Input: dimensioned drawing with shaded views. Units: mm. Origin: part minimum x, y, z. A direction names the side the tool comes from. Give positions to 0.01 mm unless a question says otherwise; leave off trailing zeros. Order: outer loops, then holes, each group sorted by start corner. A loop starts at its lowest first (then second) coordinate and runs counter-clockwise, first axis right, second up. Notation, with made-up numbers: (41.5, 57) - (84.5, 57) arc R13 cw to (84.5, 62) - close; hole circle Ø5 at (52.25, 30). An arc over 180 degrees is marked (long way). Answer as CSV lines item,"result".
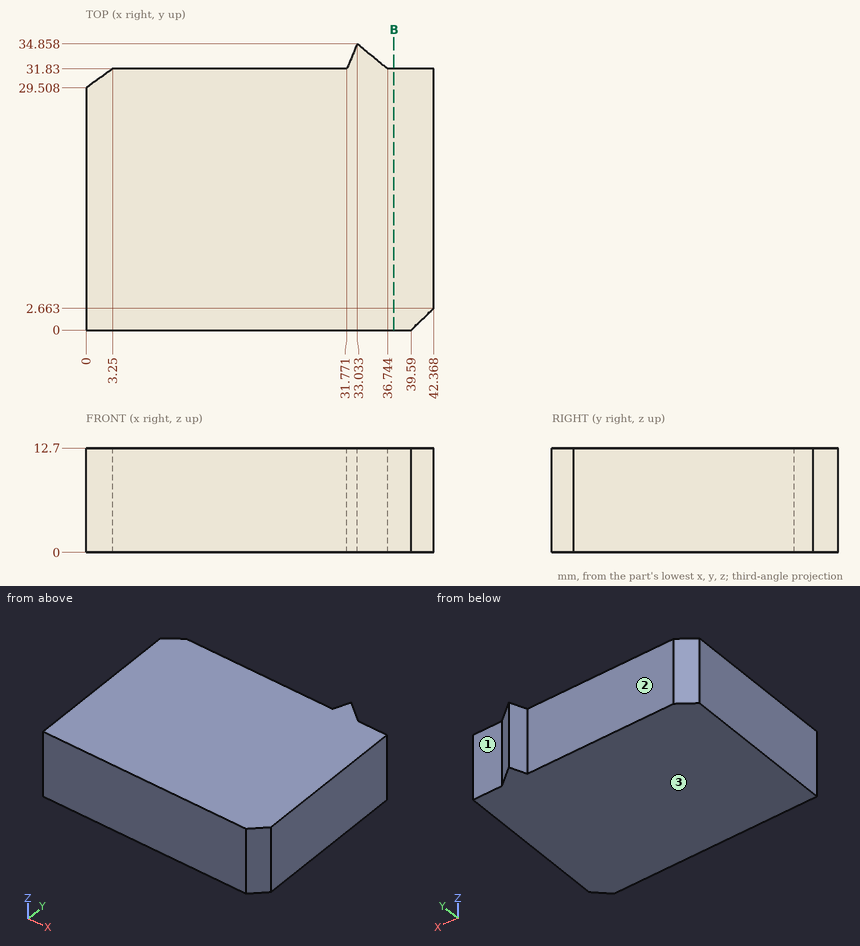
(1) Access query for the marked faces 1, 2 and 3. Directions: +Z, -Z, +X, -X, +Y, -Y. A direction counts if a zero-diameter tool reaches every point of the face in a straight line with its end or side. Return the directions, or none.
Completed:
face 1,"+Z, -Z, +X, +Y"
face 2,"+Z, -Z, -X, +Y"
face 3,"-Z, +X, -X, +Y, -Y"
(2) Contact query for flat-ended pins moving along their axis: pin 1 (2 mm diameter, centred on x = 30, z = 4.5, fed in from +Y); pin 2 (12 mm diameter, centred on x = 9.5, y = 18.5, fed in from -Z). Output: stop coordinate, or through.
Completed:
pin 1,"y = 31.83"
pin 2,"z = 0"
(3) Cut plane B-B (x = 37.5). Return loops of the section in (y, z), then the cut area to 3 significant figures.
Completed:
outline,"(0, 0) - (31.83, 0) - (31.83, 12.7) - (0, 12.7) - close"
area,"404 mm²"
(4) Ray query, line 1 (Y direction, x = 39, z = 10.25); line 2 (Y direction, x = 35, z = 7.5) (1 decimal); line 3 (X direction, y = 31.5, z = 4.25) (1 decimal). Return the intervals inside material, ascending. Write a range as from..to.
Completed:
line 1,"0..31.83"
line 2,"0..33.3"
line 3,"2.8..42.4"
